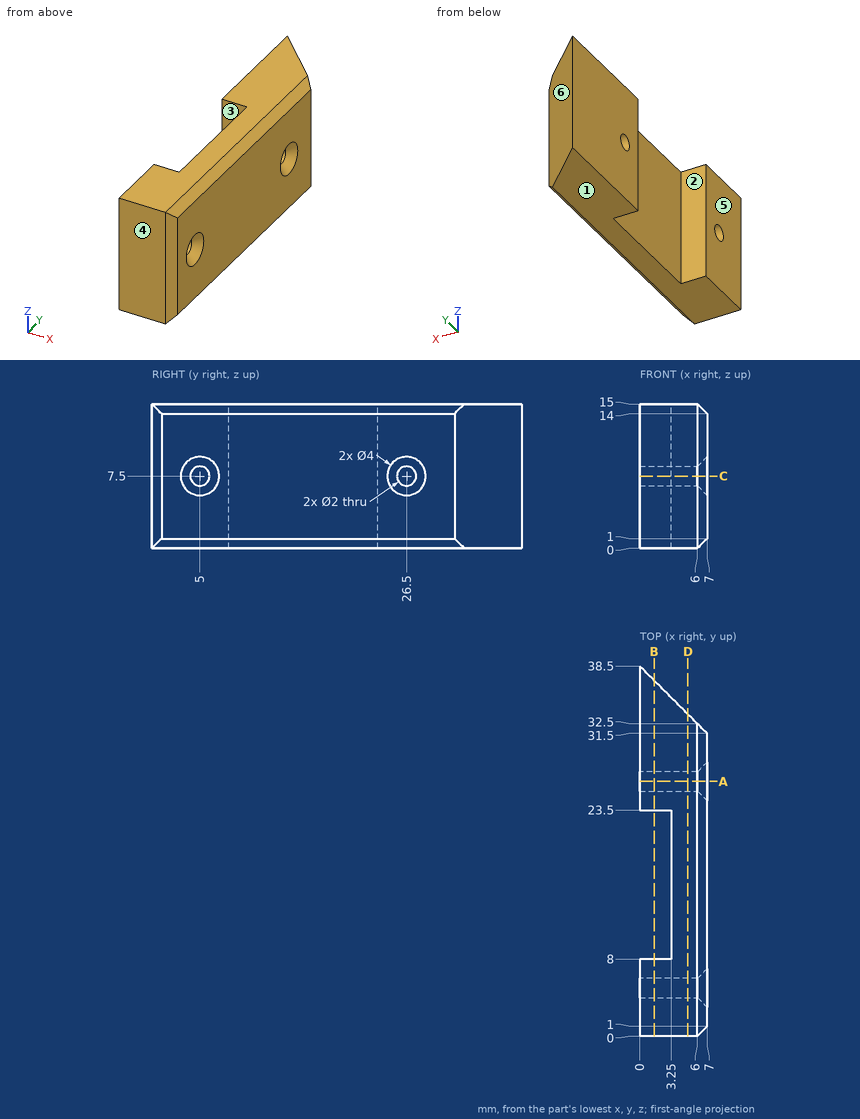
Geometry: see drawing. Coordinates: mm, zero at the bounding-box minimum. A direction names the side the tool comes from. Round coordinates to 2 decimals unless told otherwise and drop trailing zeros. Loops run counter-clockwise (first coordinate to the right, second up) from the corner with the lowest first, then second, coordinate; pieces in that order, holes last. Notation, with made-up numbers: (73, 73.5) - (77, 73.5) arc R15 cw to (77, 89.5) - close; hole circle Ø6 at (80.5, 23.5). An arc over 180 degrees is marked (long way). Use CSV: the item, a comma, the result in double quotes.
Q1. Ray query, line 1 along Z through (x, y) = (2.7, 5); line 2 along X through (y, z) = (17.5, 13.5); line 3 along Y through (x, z) = (2.75, 13.25). Return the intervals inside material, ascending.
Reported:
line 1,"0 to 6.5, 8.5 to 15"
line 2,"3.25 to 7"
line 3,"0 to 8, 23.5 to 35.75"
Q2. Mould query, pull axis Y, two halves, no side actions, for the marked faces 3, 4, 5 and 6. Classes: pulls with the +Y half, pulls with the -Y half, needs draft (parallel to the pull), parting line crosses it, or undercut.
Reported:
face 3,"undercut"
face 4,"pulls with the -Y half"
face 5,"needs draft"
face 6,"pulls with the +Y half"
Q3. Section query C-C, the plane z = 7.5. Output: boundary loops of the cut face in (x, y).
Reported:
outline,"(0, 0) - (6, 0) - (7, 1) - (7, 3) - (6, 4) - (0, 4) - close; (0, 6) - (6, 6) - (7, 7) - (7, 24.5) - (6, 25.5) - (0, 25.5) - (0, 23.5) - (3.25, 23.5) - (3.25, 8) - (0, 8) - close; (0, 27.5) - (6, 27.5) - (7, 28.5) - (7, 31.5) - (0, 38.5) - close"
Q4. Section query A-A, the plane y = 26.5. Output: boundary loops of the cut face in (x, z).
Reported:
outline,"(0, 0) - (6, 0) - (7, 1) - (7, 5.5) - (6, 6.5) - (0, 6.5) - close; (0, 8.5) - (6, 8.5) - (7, 9.5) - (7, 14) - (6, 15) - (0, 15) - close"
Q5. Reachability of the marked faces 1 and 2 from +Z, -Z, +X, -X, +Y, -Y: full face, straight path, thin tool, end or side. Return the list, or none.
Reported:
face 1,"-Z, +X, -X, +Y, -Y"
face 2,"+Z, -Z, -X"
Q6. Section query B-B, the plane x = 1.5. Output: boundary loops of the cut face in (y, z).
Reported:
outline,"(0, 0) - (8, 0) - (8, 15) - (0, 15) - close; (23.5, 0) - (37, 0) - (37, 15) - (23.5, 15) - close; hole circle Ø2 at (5, 7.5); hole circle Ø2 at (26.5, 7.5)"
Q7. Pin query (flat end, axial travel): pin 1 Ø2.5 at (y, z) = (26.5, 7.5) entering from +X; pin 2 Ø1 at (y, z) = (9.5, 11.5) entering from -X; pin 3 Ø1.2 at (y, z) = (5, 7.5) entering from +X; pin 4 Ø1.6 at (x, z) = (1.5, 5) entering from +Y. Return the tip coordinate at first contact, or that it passes through.
Reported:
pin 1,"x = 6.25"
pin 2,"x = 3.25"
pin 3,"through"
pin 4,"y = 37.8"
Q8. Section query D-D, the plane x = 5. Output: boundary loops of the cut face in (y, z), then the cut area to 3 significant figures.
Reported:
outline,"(0, 0) - (33.5, 0) - (33.5, 15) - (0, 15) - close; hole circle Ø2 at (5, 7.5); hole circle Ø2 at (26.5, 7.5)"
area,"496 mm^2"
